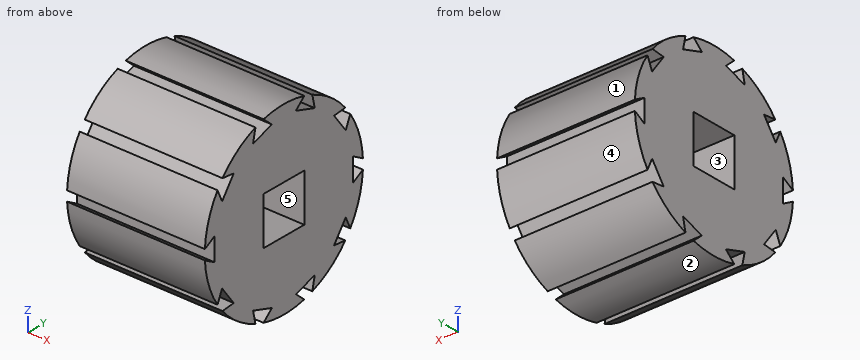
Autodesk Inventor part; units mm, degrees
ref_plane "YZ Plane" through (0, 0, 0) normal (1, 0, 0) x (0, 1, 0)
ref_plane "XZ Plane" through (0, 0, 0) normal (0, 1, 0) x (-1, 0, 0)
ref_plane "XY Plane" through (0, 0, 0) normal (0, 0, 1) x (1, 0, 0)
sketch "Sketch1" plane through (0, 0, 0) normal (1, 0, 0) x (0, 1, 0)
  circle A0 centre (0, 0) radius 50.8
  line L0 (13.081, 13.081) -> (-13.081, 13.081)
  line L1 (-13.081, 13.081) -> (-13.081, -13.081)
  line L2 (-13.081, -13.081) -> (13.081, -13.081)
  line L3 (13.081, -13.081) -> (13.081, 13.081)
  point P0 (50.7268, 2.7261)
  point P1 (50.7268, -2.7261)
  dimension "d1" = 26.162
  dimension "d2" = 26.162
extrude "Extrusion2" add sketch "Sketch1" along normal blind 76.2
sketch "Sketch2" plane through (76.2, 0, 0) normal (1, 0, 0) x (0, 0, -1)
  line L0 (-6.35, 44.45) -> (-2.7261, 50.7268)
  line L1 (6.35, 44.45) -> (-6.35, 44.45)
  line L2 (-6.35, 44.45) -> (6.35, 44.45)
  line L3 (6.35, 44.45) -> (2.7261, 50.7268)
  line L4 (-6.35, 44.45) -> (-2.7261, 50.7268)
  arc A0 (2.7261, 50.7268) -> (-2.7261, 50.7268) centre (0, 0) ccw
extrude "Extrusion3" cut sketch "Sketch2" against normal blind 76.2
pattern_circular "Circular Pattern1" count 10 over 360 about axis through (0, 0, 0) along (1, 0, 0) of "Extrusion3"
sketch "Sketch3" plane through (76.2, 0, 0) normal (1, 0, 0) x (0, 0, -1)
  point P0 (0, 0)
properties part number "220525 Large Rod Notched"
Input: part model. Units: mm. Frame: model coordinates. Face numbers are marked on the shaded views. A direction names the side the tool comes from. Coordinates: 2 decimals unless noted, no trailing zeros. Loops run counter-clockwise (first coordinate to the right, second up) from the corner with the lowest first, then second, coordinate; pieces in that order, holes last. Notation, with made-up numbers: M -12.5,18 L 38.5,18 A14 ccw 38.5,36 Z; hole C 24.5,1.25 d11. An arc over 180 degrees is marked long. Use a Markdown table: item, result. Add a question column.
1) Section D-D, the plane y = -37.5. Return the cut outline in (x, z), plus the area to 3 significant figures.
2) Section C-C, the plane y = -3. Return the cut outline in (x, z).
3) Pin query (flat end, axial travel): P1, Ø1.5, axis at x = 43.5, y = 27, coming from the -Z side; P2, Ø6, axis at x = 53, y = -36, coming from the +Z side. Return the tip coordinate at first contact, or that it passes through.
4) Draft query along Y for the marked faces 1, 2 and 3. Return one class per face: +Y half, -Y half, draft (parallel to the pull), parting line (faces both ways), or undercut.
5) Section B-B, the plane y = 35. Return the cut outline in (x, z), plus the area to 3 significant figures.
6) Set-up query: the marked faces 4 and 5. Return all of +Z, -Z, +X, -X, +Y, -Y with unobstructed straight access to the full face (end or side cutting, diameter ignored); none if empty.
7) Line query: L1, parallel to Z at x = 54, y = 9; L2, parallel to Y at x = 30.5, z = 2.5; L3, parallel to Y at x = 65, z = 3. Output: solid intervals per line, ascending. Write a range as from..to.
8) Section A-A, the plane z = -0.5. Return the cut outline in (x, y), plus the area to 3 significant figures.
Answer below:
| question | item | result |
|---|---|---|
| 1 | outline | M 0,-34.27 L 76.2,-34.27 L 76.2,-31.82 L 0,-31.82 Z; M 0,-24.01 L 76.2,-24.01 L 76.2,24.01 L 0,24.01 Z; M 0,31.82 L 76.2,31.82 L 76.2,34.27 L 0,34.27 Z |
| 1 | area | 4,030 mm2 |
| 2 | outline | M 0,-50.71 L 76.2,-50.71 L 76.2,-13.08 L 0,-13.08 Z; M 0,13.08 L 76.2,13.08 L 76.2,50.71 L 0,50.71 Z |
| 3 | P1 | z = -43.49 |
| 3 | P2 | z = 38.62 |
| 4 | face 1 | +Y half |
| 4 | face 2 | parting line |
| 4 | face 3 | undercut |
| 5 | outline | M 0,-36.82 L 76.2,-36.82 L 76.2,-31.56 L 0,-31.56 Z; M 0,-27.45 L 76.2,-27.45 L 76.2,27.45 L 0,27.45 Z; M 0,31.56 L 76.2,31.56 L 76.2,36.82 L 0,36.82 Z |
| 5 | area | 4,990 mm2 |
| 6 | face 4 | -Z, +X, -X, +Y |
| 6 | face 5 | +X, -X |
| 7 | L1 | -50..-45.41, -43.81..-13.08, 13.08..43.81, 45.41..50 |
| 7 | L2 | -44.45..-13.08, 13.08..44.45 |
| 7 | L3 | -50.71..-50.25, -44.45..-13.08, 13.08..44.45, 50.25..50.71 |
| 8 | outline | M 0,-44.45 L 76.2,-44.45 L 76.2,-13.08 L 0,-13.08 Z; M 0,13.08 L 76.2,13.08 L 76.2,44.45 L 0,44.45 Z |
| 8 | area | 4,780 mm2 |
